Autodesk Inventor part; units mm, degrees
ref_plane "YZ Plane" through (0, 0, 0) normal (1, 0, 0) x (0, 1, 0)
ref_plane "XZ Plane" through (0, 0, 0) normal (0, 1, 0) x (-1, 0, 0)
ref_plane "XY Plane" through (0, 0, 0) normal (0, 0, 1) x (1, 0, 0)
sketch "Sketch1" plane through (0, 0, 0) normal (0, 0, 1) x (1, 0, 0)
  line L0 (0, 0) -> (0, 10)
  line L1 (6.245, 10) -> (6.245, 7)
  circle A0 centre (3.1225, 12.5) radius 2.5
  arc A1 (6.245, 10) -> (0, 10) centre (3.1225, 12.5) ccw
  line L2 (6, 10) -> (0, 10) construction
  line L3 (8, 0) -> (8, 7)
  line L4 (8, 7) -> (6.245, 7)
  line L5 (0, 0) -> (8, 0)
  dimension "d2" = 8
  dimension "d3" = 5
  dimension "d5" = 10
  dimension "d17" = 7
  dimension "d18" = 3
  dimension "d19" = 8
extrude "Extrusion1" add sketch "Sketch1" along normal blind 20
sketch "Sketch2" plane through (0, 0, 0) normal (-1, 0, 0) x (0, 0, 1)
  point P0 (0, 0)
sketch "Sketch3" plane through (6.245, 0, 0) normal (1, 0, 0) x (0, 0, -1)
  line L0 (0, 10) -> (-20, 10)
  line L1 (-17.5032, 10) -> (-17.5032, 16.6156)
  line L2 (-17.5032, 16.6156) -> (-2.428, 16.6156)
  line L3 (0, 16.5) -> (-20, 16.5)
  line L4 (-2.428, 16.6156) -> (-2.428, 10)
  line L5 (-2.428, 10) -> (-17.5032, 10)
  point P0 (0, 0)
extrude "Extrusion2" cut sketch "Sketch3" along normal mid plane 20
sketch "Sketch4" plane through (6.245, 0, 0) normal (1, 0, 0) x (0, 0, -1)
  line L0 (0, 0) -> (-20, 0)
  line L1 (0, 0) -> (0, 10)
  line L2 (-20, 0) -> (0, 0)
  line L3 (0, 0) -> (0, 6.4437)
  line L4 (0, 6.4437) -> (-20, 6.4437)
  line L5 (-20, 6.4437) -> (-20, 0)
extrude "Extrusion3" add sketch "Sketch4" along normal blind 0.1
sketch "Sketch5" plane through (6.245, 10, 17.5032) normal (1, 0, 0) x (0, 0, -1)
  line L0 (0, 6.5) -> (0, 0)
  line L1 (0, 6.5) -> (0, -1.5)
  line L2 (0, -1.5) -> (15.0752, -1.5)
  line L3 (15.0752, 6.5) -> (15.0752, -1.5)
  line L4 (0, 6.5) -> (15.0752, 6.5)
  point P0 (17.5032, -10)
  dimension "d12" = 8
  dimension "d13" = 15.0752
extrude "Extrusion4" cut sketch "Sketch5" against normal blind 10
fillet "Fillet1" radius 2 1 edges at (6.245, 8.5, 9.9656)
fillet "Fillet2" radius 2 1 edges at (0, 8.5, 9.9656)
sketch "Sketch6" plane through (8, 0, 0) normal (1, 0, 0) x (0, 0, -1)
  line L0 (-2.428, 7) -> (-2.428, 10)
  line L1 (-2.428, 10) -> (-17.5032, 10)
  line L2 (-17.5032, 18.1901) -> (-2.428, 18.1901)
  line L3 (0, 10) -> (-2.428, 10)
  line L4 (-2.428, 18.1901) -> (-2.428, 10)
  line L5 (-17.5032, 10) -> (-17.5032, 10)
  line L6 (-17.5032, 18.1901) -> (-17.5032, 10)
  point P0 (0, 0)
  point P1 (-17.5032, 16.5)
extrude "Extrusion5" cut sketch "Sketch6" against normal blind 10
properties part number "HingeBase1"
The model under review builds one solid part; all positions refer to its coordinate system, in mm. A direction names the side the tool comes from. Round coordinates to 2 decimals unless told otherwise and drop trailing zeros. Write each loop counter-clockwise with the first axis right and the second up, starting at its lowest first coordinate (ties: lowest second). Pieces come first, ordered by that corner, then holes. Notation, with made-up numbers: (88.5, -9) - (137.5, -9) arc R23 cw to (137.5, 4) - close; hole circle Ø10 at (69, 43). An arc over 180 degrees is marked (long way). Use one line per item in the form item = value.
Q1. Consider section A-A (y = 9.75). State the section outline as (x, z) points (3 decimals).
Answer key:
outline = (0, 0) - (6.245, 0) - (6.245, 2.428) - (0, 2.428) - close; (0, 17.503) - (6.245, 17.503) - (6.245, 20) - (0, 20) - close
Q2. Consider section D-D (z = 15.5). State the section outline as (x, y) points (1 decimal).
Answer key:
outline = (0, 0) - (8, 0) - (8, 7) - (6.2, 7) arc R2 ccw to (4.3, 8.5) - (2, 8.5) arc R2 ccw to (0, 6.5) - close
Q3. Tool access review of faces 1 (the cylindrical face through (0.6, 7.93, 10.07)), 2 (the cylindrical face through (5.55, 8.07, 10.07)), 3 (the flat face through (3, 8.5, 10)), 4 (the flat face through (6.245, 9, 19)): name each direction out of +Z, -Z, +X, -X, +Y, -Y from which nothing blocks a thin tool from reaching the whole face with its end or side.
Answer key:
face_1 = -X, +Y
face_2 = +X, +Y
face_3 = +X, -X, +Y
face_4 = +Z, -Z, +X
Q4. For line 1 (Z direction, x = 7, y = 11.75); line 2 (Y direction, x = 3.5, z = 13.25); line 3 (X direction, y = 13.75, z = 19.25), list the stretches that pass through material, from the lowest coordinate up. Write a range as [from, to].
Answer key:
line_1 = [0, 2.43], [17.5, 20]
line_2 = [0, 8.5]
line_3 = [-0.68, 0.96], [5.29, 6.92]
Q5. Insertion check: pin 1 Ø1.9 at (x, z) = (7, 13.5) entering from +Y; pin 2 Ø4.5 at (x, y) = (3.12, 12.5) entering from -Z; pin 3 Ø2.5 at (y, z) = (8.5, 0.5) entering from +X (3 decimals); pin 4 Ø2.5 at (x, z) = (3.5, 12) entering from +Y. Each pin has a flat end and moves straight along its axis. Give the tip position at first contact, or say it passes through.
Answer key:
pin_1 = 7.48
pin_2 = through
pin_3 = 6.245
pin_4 = 8.5
Q6. Draft analysis for pull direction X (two halves, no side actions). For faces 5 (the cylindrical face through (2.58, 14.94, 1.2)), 6 (the flat face through (0, 4, 10)), 7 (the cylindrical face through (3, 16.5, 1.2)), state which applies: +X half, -X half, draft (parallel to the pull), parting line (faces both ways), or undercut.
Answer key:
face_5 = undercut
face_6 = -X half
face_7 = parting line
Q7. Consider section B-B (z = 17.75). State the section outline as (x, y) points (1 decimal), and give its area (3 significant figures).
Answer key:
outline = (0, 0) - (8, 0) - (8, 7) - (6.2, 7) - (6.2, 10) arc R4 ccw (long way) to (0, 10) - close; hole circle Ø5 at (3.1, 12.5)
area = 98.8 mm2
Q8. Consider section C-C (x = 3.25). State the section outline as (y, z) points.
Answer key:
outline = (0, 0) - (10, 0) - (10, 2.43) - (8.5, 2.43) - (8.5, 17.5) - (10, 17.5) - (10, 20) - (0, 20) - close; (15, 0) - (16.5, 0) - (16.5, 2.43) - (15, 2.43) - close; (15, 17.5) - (16.5, 17.5) - (16.5, 20) - (15, 20) - close
